from build123d import *

# Parameters (mm, degrees)
PAD_DEPTH    = 3
SKETCH001_R  = 2.5
POCKET_DEPTH = 5


with BuildPart() as part:
    # Sketch → Pad (new body)
    with BuildSketch(Plane.XY):
        with BuildLine():
            Line((-8.15, 40), (-8.15, -40))
            Line((-8.15, -40), (8.15, -40))
            Line((8.15, -40), (8.15, -8.35))
            ThreePointArc((8.15, -8.35), (16.5, 0), (8.15, 8.35))
            Line((8.15, 8.35), (8.15, 40))
            Line((8.15, 40), (-8.15, 40))
        make_face()
    extrude(amount=PAD_DEPTH)

    # Sketch001 (on Face8 of Pad) → Pocket (cut)
    with BuildSketch(Plane.XY.offset(3)):
        with Locations((0, 25)):
            Circle(SKETCH001_R)
        with Locations((0, -25)):
            Circle(SKETCH001_R)
    extrude(amount=-POCKET_DEPTH, mode=Mode.SUBTRACT)


solid = part.part
Here's how the part is built. I have some questions about the finished solid (model axes, mm). A direction names the side the tool comes from. Give positions to 0.01 mm unless a question says otherwise; leave off trailing zeros. Write each loop counter-clockwise with the first axis right and the second up, starting at its lowest first coordinate (ties: lowest second). Pieces come first, ordered by that corner, then holes. Notation, with made-up numbers: (10.5, 48.5) -> (65.5, 48.5) arc R20 cw to (65.5, 72.5) -> close; hole circle Ø4 at (-19.5, -13.75). An arc over 180 degrees is marked (long way). Use one line per item in the form item = value. Start each with the question number.
1. Imagine slicing it at B-B on y = -25. List the corners of the cut face in (x, z) for me.
2. On a 3-axis mill with a long thin cutter (end or side, diameter ignored), from which of +Z, -Z, +X, -X, +Y, -Y can I reach the whole of each face in a straight line? I mean faces 1 (the face through (8.15, 24, 1)), 2 (the face through (1, 1, 0)). Say none if no direction works.
3. If I drill on L1, parallel to Y at x = 0, z = 1.9; L2, parallel to Y at x = 2.25, z = 0.75; L3, parallel to X at y = -34, z = 1.6, over which ranges is the centre line in solid material (lowest first)?
4. Imagine slicing it at D-D on y = -5. List the corners of the cut face in (x, z) for me.
5. Thinking about a two-plate mould opening in Y: for faces 3 (the face through (0, -40, 1)), 4 (the face through (8.15, -24, 1)), 5 (the face through (-0.33, -22.52, 1.52)), which applies, +Y half, -Y half, draft (parallel to the pull), parting line (faces both ways), or undercut?
6. Imagine slicing it at C-C on x = 15. List the corners of the cut face in (y, z) for me, plus the area to 3 significant figures.
7. Will this pin go through, and if not, where does the flat tip stop? pin 1 Ø0.9 at (y, z) = (19.5, 1) entering from +X.
8. Imagine slicing it at A-A on z = 1.55. List the corners of the cut face in (x, y) for me.
Entries:
q1.outline = (-8.15, 0) -> (-2.5, 0) -> (-2.5, 3) -> (-8.15, 3) -> close; (2.5, 0) -> (8.15, 0) -> (8.15, 3) -> (2.5, 3) -> close
q2.face_1 = +Z, -Z, +X, +Y
q2.face_2 = -Z, +X, -X, +Y, -Y
q3.L1 = -40 to -27.5, -22.5 to 22.5, 27.5 to 40
q3.L2 = -40 to -26.09, -23.91 to 23.91, 26.09 to 40
q3.L3 = -8.15 to 8.15
q4.outline = (-8.15, 0) -> (14.84, 0) -> (14.84, 3) -> (-8.15, 3) -> close
q5.face_3 = -Y half
q5.face_4 = draft
q5.face_5 = undercut
q6.outline = (-4.77, 0) -> (4.77, 0) -> (4.77, 3) -> (-4.77, 3) -> close
q6.area = 28.6 mm²
q7.pin_1 = 8.15
q8.outline = (-8.15, -40) -> (8.15, -40) -> (8.15, -8.35) arc R8.35 ccw to (8.15, 8.35) -> (8.15, 40) -> (-8.15, 40) -> close; hole circle Ø5 at (0, -25); hole circle Ø5 at (0, 25)
